```python
from build123d import *

# Parameters (mm, degrees)
CROQUIS1_R              = 12
SALIENTE_EXTRUIR1_DEPTH = 69
CROQUIS2_R              = 12
CROQUIS2_W              = 13
CROQUIS2_H              = 4.5
SALIENTE_EXTRUIR2_DEPTH = 25


with BuildPart() as part:
    # Croquis1 → Saliente-Extruir1 (new body)
    with BuildSketch(Plane.XY):
        Circle(CROQUIS1_R)
    extrude(amount=SALIENTE_EXTRUIR1_DEPTH)

    # Croquis2 → Saliente-Extruir2 (add)
    with BuildSketch(Plane.XY.offset(69)):
        Circle(CROQUIS2_R)
        with Locations((0, -1.565571557)):
            Rectangle(CROQUIS2_W, CROQUIS2_H, mode=Mode.SUBTRACT)
    extrude(amount=SALIENTE_EXTRUIR2_DEPTH)


solid = part.part
```
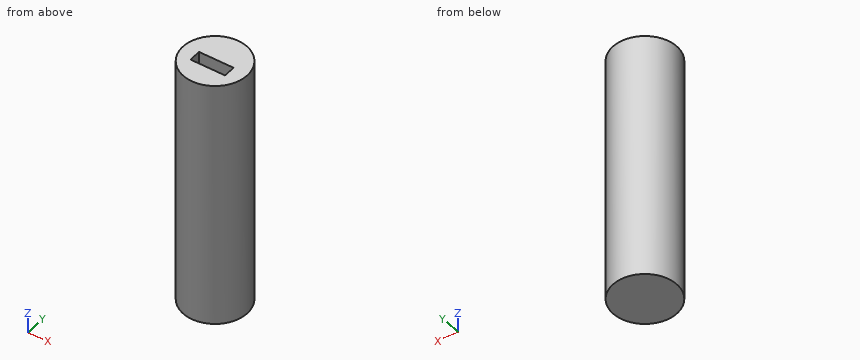
Source: CAD feature listing. Evaluate the final solid. Frame: model axes, mm. Coordinates: 2 decimals unless noted, no trailing zeros. Write each loop counter-clockwise with the first axis right and the second up, starting at its lowest first coordinate (ties: lowest second). Pieces come first, ordered by that corner, then holes. Notation, with made-up numbers: (-19, 88) - (31, 88) arc R21 cw to (31, 96) - close; hole circle Ø7 at (-10.5, 77). An arc over 180 degrees is marked (long way). Answer as a JSON object with one key per item and string values.
Q1. Section query C-C, the plane z = 8.5. Output: boundary loops of the cut face in (x, y).
Ans:
{"outline": "circle Ø24 at (0, 0)"}
Q2. First-contact query: pin 1 Ø2 at (y, z) = (-2.5, 79) entering from -X; pin 2 Ø3.5 at (x, y) = (-3, -1.5) entering from +Z; pin 3 Ø1.5 at (y, z) = (-9, 15) entering from +X. Flat tips, straight axial feed; report the tip coordinate or a pass-through.
Ans:
{"pin 1": "stops at x = -11.91", "pin 2": "stops at z = 69", "pin 3": "stops at x = 8.71"}
Q3. Section query B-B, the plane y = -1.5. Output: boundary loops of the cut face in (x, z), plus the area to 3 significant figures.
Ans:
{"outline": "(-11.91, 0) - (11.91, 0) - (11.91, 94) - (6.5, 94) - (6.5, 69) - (-6.5, 69) - (-6.5, 94) - (-11.91, 94) - close", "area": "1,910 mm2"}
Q4. Section query A-A, the plane x = 0. Output: boundary loops of the cut face in (y, z).
Ans:
{"outline": "(-12, 0) - (12, 0) - (12, 94) - (0.68, 94) - (0.68, 69) - (-3.82, 69) - (-3.82, 94) - (-12, 94) - close"}
Q5. Section query D-D, the plane x = -9.75. Output: boundary loops of the cut face in (y, z).
Ans:
{"outline": "(-7, 0) - (7, 0) - (7, 94) - (-7, 94) - close"}
Q6. Material intervals for line 1 (Z direction, x = 1, y = -1.5); line 2 (Y direction, x = 5, z = 85); line 3 (Y direction, x = 4, z = 87.5), sorted ascending. Write a range as [from, to].
Ans:
{"line 1": "z = [0, 69]", "line 2": "y = [-10.91, -3.82], [0.68, 10.91]", "line 3": "y = [-11.31, -3.82], [0.68, 11.31]"}
